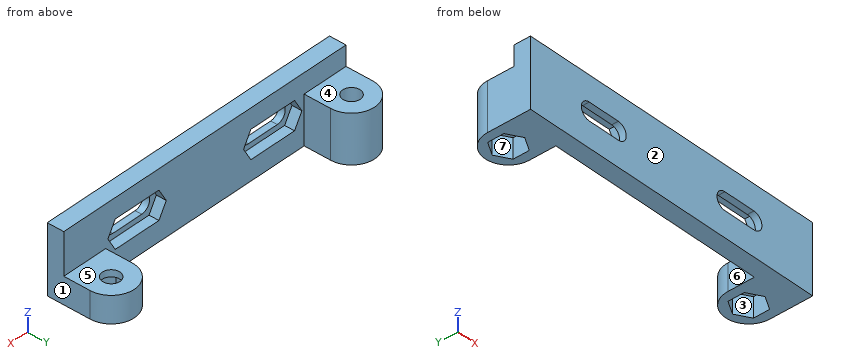
Autodesk Inventor part; units mm, degrees
ref_plane "YZ Plane" through (0, 0, 0) normal (1, 0, 0) x (0, 1, 0)
ref_plane "XZ Plane" through (0, 0, 0) normal (0, 1, 0) x (-1, 0, 0)
ref_plane "XY Plane" through (0, 0, 0) normal (0, 0, 1) x (1, 0, 0)
sketch "Skizze1" plane through (0, 0, 0) normal (0, 0, 1) x (1, 0, 0)
  circle A0 centre (7, 13) radius 2.65
  circle A1 centre (87.334, 13) radius 2.65
  arc A2 (14, 13) -> (0, 13) centre (7, 13) ccw
  arc A3 (94.334, 13) -> (80.334, 13) centre (87.334, 13) ccw
  line L0 (94.334, 0) -> (0, 0)
  line L1 (0, 5) -> (94.334, 5)
  line L2 (94.334, 13) -> (94.334, 0)
  line L3 (80.334, 13) -> (80.334, 5)
  line L4 (14, 13) -> (14, 5)
  line L5 (0, 13) -> (0, 0)
  dimension "d4" = 5.3
  dimension "d5" = 5.3
  dimension "d8" = 80.334
  dimension "d18" = 5
  dimension "d21" = 7
  dimension "d22" = 13
extrude "Extrusion1" add sketch "Skizze1" along normal blind 12.5 and the other way blind 8 contours L1 L2 L0 L5
extrude "Extrusion2" add sketch "Skizze1" against normal blind 8 contours L3 A3 L2 L1
extrude "Extrusion3" add sketch "Skizze1" along normal blind 6.5 and the other way blind 8 contours L4 L1 L5 A2
sketch "Skizze2" plane through (0, 0, -8) normal (0, 0, -1) x (-1, 0, 0)
  circle A0 centre (-87.334, 13) radius 2.65
  circle A1 centre (-7, 13) radius 2.65
  line L0 (-87.334, 17.9075) -> (-83.084, 15.4537)
  line L1 (-83.084, 15.4537) -> (-83.084, 10.5463)
  line L2 (-83.084, 10.5463) -> (-87.334, 8.0925)
  line L3 (-87.334, 8.0925) -> (-91.584, 10.5463)
  line L4 (-91.584, 10.5463) -> (-91.584, 15.4537)
  line L5 (-91.584, 15.4537) -> (-87.334, 17.9075)
  line L6 (-7, 17.9075) -> (-2.75, 15.4537)
  line L7 (-2.75, 15.4537) -> (-2.75, 10.5463)
  line L8 (-2.75, 10.5463) -> (-7, 8.0925)
  line L9 (-7, 8.0925) -> (-11.25, 10.5463)
  line L10 (-11.25, 10.5463) -> (-11.25, 15.4537)
  line L11 (-11.25, 15.4537) -> (-7, 17.9075)
  point P0 (0, 0)
  dimension "d23" = 8.5
  dimension "d24" = 8.5
extrude "Extrusion4" cut sketch "Skizze2" against normal blind 6 contours L0 L1 L2 L3 L4 L5
extrude "Extrusion5" cut sketch "Skizze2" against normal blind 6 contours A1 | L6 L7 L8 L9 L10 L11
sketch "Skizze3" plane through (0, 0, 12.5) normal (0, -1, 0) x (1, 0, 0)
  line L0 (94.334, 0) -> (94.334, -20.5)
  line L1 (0, 0) -> (94.334, 0)
  line L2 (0, -20.5) -> (0, 0)
  line L3 (94.334, -20.5) -> (0, -20.5)
  line L4 (0, -20.5) -> (0, 0)
  line L5 (0, -10.25) -> (94.334, -10.25) construction
  line L6 (94.334, 0) -> (94.334, -20.5)
  line L7 (17, -10.25) -> (32, -10.25) construction
  line L8 (19.65, -12.9) -> (29.35, -12.9)
  line L9 (29.35, -7.6) -> (19.65, -7.6)
  arc A0 (19.65, -7.6) -> (19.65, -12.9) centre (19.65, -10.25) ccw
  arc A1 (29.35, -12.9) -> (29.35, -7.6) centre (29.35, -10.25) ccw
  line L10 (62.334, -10.25) -> (77.334, -10.25) construction
  line L11 (64.984, -12.9) -> (74.684, -12.9)
  line L12 (74.684, -7.6) -> (64.984, -7.6)
  arc A2 (64.984, -7.6) -> (64.984, -12.9) centre (64.984, -10.25) ccw
  arc A3 (74.684, -12.9) -> (74.684, -7.6) centre (74.684, -10.25) ccw
  point P0 (0, -12.5)
  point P1 (24.5, -10.25)
  point P2 (69.834, -10.25)
  dimension "d34" = 5.3
  dimension "d35" = 5.3
  dimension "d36" = 15
  dimension "d37" = 15
  dimension "d38" = 17
  dimension "d39" = 17
extrude "Extrusion6" cut sketch "Skizze3" against normal through all contours A0 L9 A1 L8 | A2 L12 A3 L11
sketch "Skizze4" plane through (0, 5, 12.5) normal (0, 1, 0) x (1, 0, 0)
  line L0 (74.684, 7.6) -> (64.984, 7.6)
  arc A0 (64.984, 12.9) -> (64.984, 7.6) centre (64.984, 10.25) ccw
  line L1 (64.984, 12.9) -> (74.684, 12.9)
  arc A1 (74.684, 7.6) -> (74.684, 12.9) centre (74.684, 10.25) ccw
  line L2 (29.35, 7.6) -> (19.65, 7.6)
  arc A2 (19.65, 12.9) -> (19.65, 7.6) centre (19.65, 10.25) ccw
  line L3 (19.65, 12.9) -> (29.35, 12.9)
  arc A3 (29.35, 7.6) -> (29.35, 12.9) centre (29.35, 10.25) ccw
  line L4 (14, 6) -> (0, 6)
  line L5 (0, 6) -> (0, 0)
  line L6 (94.334, 0) -> (0, 0)
  line L7 (94.334, 12.5) -> (94.334, 0)
  line L8 (94.334, 12.5) -> (80.334, 12.5)
  line L9 (80.334, 12.5) -> (80.334, 20.5)
  line L10 (14, 20.5) -> (80.334, 20.5)
  line L11 (14, 20.5) -> (14, 6)
  line L12 (77.1378, 6) -> (72.2303, 6)
  line L13 (72.2303, 6) -> (69.7765, 10.25)
  line L14 (69.7765, 10.25) -> (72.2303, 14.5)
  line L15 (72.2303, 14.5) -> (77.1378, 14.5)
  line L16 (77.1378, 14.5) -> (79.5915, 10.25)
  line L17 (79.5915, 10.25) -> (77.1378, 6)
  line L18 (62.5303, 6) -> (60.0765, 10.25)
  line L19 (60.0765, 10.25) -> (62.5303, 14.5)
  line L20 (62.5303, 14.5) -> (67.4378, 14.5)
  line L21 (67.4378, 14.5) -> (69.8915, 10.25)
  line L22 (69.8915, 10.25) -> (67.4378, 6)
  line L23 (67.4378, 6) -> (62.5303, 6)
  line L24 (31.8037, 6) -> (26.8963, 6)
  line L25 (26.8963, 6) -> (24.4425, 10.25)
  line L26 (24.4425, 10.25) -> (26.8963, 14.5)
  line L27 (26.8963, 14.5) -> (31.8037, 14.5)
  line L28 (31.8037, 14.5) -> (34.2575, 10.25)
  line L29 (34.2575, 10.25) -> (31.8037, 6)
  line L30 (17.1963, 6) -> (14.7425, 10.25)
  line L31 (14.7425, 10.25) -> (17.1963, 14.5)
  line L32 (17.1963, 14.5) -> (22.1037, 14.5)
  line L33 (22.1037, 14.5) -> (24.5575, 10.25)
  line L34 (24.5575, 10.25) -> (22.1037, 6)
  line L35 (22.1037, 6) -> (17.1963, 6)
  line L36 (72.2303, 6) -> (67.4378, 6)
  line L37 (74.684, 7.6) -> (64.984, 7.6)
  line L38 (72.2303, 14.5) -> (67.4378, 14.5)
  line L39 (26.8963, 6) -> (22.1037, 6)
  line L40 (26.8963, 14.5) -> (22.1037, 14.5)
  point P0 (0, 12.5)
  dimension "d42" = 8.5
extrude "Extrusion7" cut sketch "Skizze4" against normal blind 3 contours A1 L1 L14 L15 L16 L17 L12 L13 L0 | L13 L36 L22 L0 | L22 L23 L18 L19 L20 L21 L1 A0 L0 | L1 L21 L38 L14 | A3 L3 L26 L27 L28 L29 L24 L25 L2 | L25 L39 L34 L2 | L34 L35 L30 L31 L32 L33 L3 A2 L2 | L3 L33 L40 L26
equation "\"d4\" = d5"
equation "\"d10\" = d14"
equation "\"d29\" = d14"
equation "\"d24\" = d23"
equation "\"d35\" = d34"
equation "\"d37\" = d36"
properties part number "Door_Panel" material "ABS-Kunststoff"
Verification items for the finished model (mm, model axes). Face numbers are marked on the shaded views. A direction names the side the tool comes from. Round coordinates to 2 decimals unless told otherwise and drop trailing zeros. Loops run counter-clockwise (first coordinate to the right, second up) from the corner with the lowest first, then second, coordinate; pieces in that order, holes last. Notation, with made-up numbers: (77, 87) - (110, 87) arc R18 cw to (110, 102) - close; hole circle Ø9 at (-3.75, -27). An arc over 180 degrees is marked (long way). Answer in a Markdown table with one row per item. Add a question column.
Q1. Section check A-A on x = 66. Enter the section's corners in (y, z), plus the area to 3 significant figures.
Q2. Tool access check on the marked faces 4, 5, 6 and 7. Record the directions out of +Z, -Z, +X, -X, +Y, -Y that give a thin tool (end or side, any length) a straight path to the whole face; none if there is none.
Q3. Section check C-C on z = 7.5. Enter the section's corners in (x, y), plus the area to 3 significant figures.
Q4. Material ranges on line 1 (Z direction, x = 26, y = 1.5); line 2 (X direction, y = 2.25, z = -1.5); line 3 (Y direction, x = 7, z = 0.5), recorded low to high.
Q5. Section check D-D on x = 46. Enter the section's corners in (y, z).
Q6. Section check B-B on z = -4.25. Enter the section's corners in (x, y), plus the area to 3 significant figures.
Q7. Gauge pin test, flat ends, axial feed: pin 1 (9.5 mm diameter, centred on x = 28, z = 1, fed in from +Y); pin 2 (10 mm diameter, centred on x = 23, y = 12, fed in from -Z); pin 3 (4 mm diameter, centred on y = 8, z = 2.5, fed in from +X); pin 4 (4 mm diameter, centred on x = 88, y = 12, fed in from -Z). Record the tip position at first contact, or that the pin passes through.
Q8. Release check for a two-part mould opening along X. For the marked faces 1, 2 and 3 record: pulls with the +X half, pulls with the -X half, needs draft (parallel to the pull), parting line crosses it, or undercut.
Found:
| question | item | result |
|---|---|---|
| 1 | outline | (0, -8) - (5, -8) - (5, -2) - (2, -2) - (2, -0.4) - (0, -0.4) - close; (0, 4.9) - (2, 4.9) - (2, 6.5) - (5, 6.5) - (5, 12.5) - (0, 12.5) - close |
| 1 | area | 66.4 mm² |
| 2 | face 4 | +Z, +X, -X, +Y |
| 2 | face 5 | +Z, +X, +Y |
| 2 | face 6 | +Z, -Z, +Y |
| 2 | face 7 | -Z |
| 3 | outline | (0, 0) - (94.33, 0) - (94.33, 5) - (0, 5) - close |
| 3 | area | 472 mm² |
| 4 | line 1 | z = -8 to -0.4, 4.9 to 12.5 |
| 4 | line 2 | x = 0 to 16.91, 32.09 to 62.24, 77.43 to 94.33 |
| 4 | line 3 | y = 0 to 10.35, 15.65 to 20 |
| 5 | outline | (0, -8) - (5, -8) - (5, 12.5) - (0, 12.5) - close |
| 6 | outline | (0, 0) - (94.33, 0) - (94.33, 13) arc R7 ccw to (80.33, 13) - (80.33, 5) - (14, 5) - (14, 13) arc R7 ccw to (0, 13) - close; hole (2.75, 10.55) - (7, 8.09) - (11.25, 10.55) - (11.25, 15.45) - (7, 17.91) - (2.75, 15.45) - close; hole (83.08, 10.55) - (87.33, 8.09) - (91.58, 10.55) - (91.58, 15.45) - (87.33, 17.91) - (83.08, 15.45) - close |
| 6 | area | 724 mm² |
| 7 | pin 1 | stops at y = 5 |
| 7 | pin 2 | passes through |
| 7 | pin 3 | stops at x = 14 |
| 7 | pin 4 | stops at z = -2 |
| 8 | face 1 | pulls with the +X half |
| 8 | face 2 | needs draft |
| 8 | face 3 | undercut |
